Input: part model. Units: mm. Frame: model coordinates. Face numbers are marked on the shaded views. A direction names the side the tool comes from. Coordinates: 2 decimals unless noted, no trailing zeros. Loops run counter-clockwise (first coordinate to the right, second up) from the corner with the lowest first, then second, coordinate; pieces in that order, holes last.
```python
from build123d import *

# Parameters (mm, degrees)
SKETCH1_R                = 50
BOSS_EXTRUDE1_DEPTH      = 129.45
CUT_EXTRUDE1_DEPTH       = 129.45
CUT_EXTRUDE1_DEPTH_BACK  = 129.45
SKETCH3_W                = 73.302623589
SKETCH3_H                = 112.659736925
BOSS_EXTRUDE2_DEPTH      = 10
BOSS_EXTRUDE2_DEPTH_BACK = 10
SKETCH2_R                = 15


with BuildPart() as part:
    # Sketch1 → Boss-Extrude1 (new body)
    with BuildSketch(Plane(origin=(0, 0, 0), x_dir=(0, 0, -1), z_dir=(1, 0, 0))):
        Circle(SKETCH1_R)
    extrude(amount=-BOSS_EXTRUDE1_DEPTH)

    # Sketch3 → Cut-Extrude1 (cut, two sides: drawn at the far end of the back side and taken through both)
    with BuildSketch(Plane(origin=(0, 0, 0), x_dir=(1, 0, 0), z_dir=(0, 1, 0)).offset(-CUT_EXTRUDE1_DEPTH_BACK)):
        with Locations((-96.101311794, -3.115771473)):
            Rectangle(SKETCH3_W, SKETCH3_H)
    extrude(amount=CUT_EXTRUDE1_DEPTH + CUT_EXTRUDE1_DEPTH_BACK, mode=Mode.SUBTRACT)

    # Sketch2 → Boss-Extrude2 (add, two sides: drawn at the far end of the back side and taken through both)
    with BuildSketch(Plane(origin=(0, 0, 0), x_dir=(1, 0, 0), z_dir=(0, 1, 0)).offset(-BOSS_EXTRUDE2_DEPTH_BACK)):
        with BuildLine():
            Line((-129.45, 30), (-59.45, 30))
            Line((-59.45, 30), (-59.45, -30))
            Line((-59.45, -30), (-129.45, -30))
            ThreePointArc((-129.45, -30), (-159.45, 0), (-129.45, 30))
        make_face()
        with Locations(Location((-129.45, 0, 0), (0, 0, 270))):
            Circle(SKETCH2_R, mode=Mode.SUBTRACT)
    extrude(amount=BOSS_EXTRUDE2_DEPTH + BOSS_EXTRUDE2_DEPTH_BACK)


solid = part.part
```
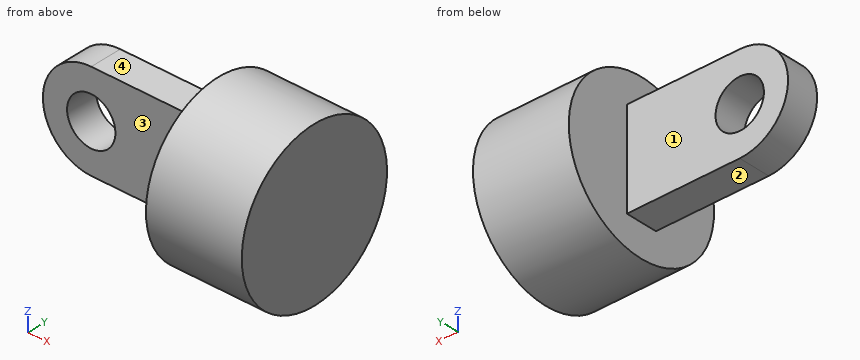
Item 1: Section query C-C (x = -34.5). Output: boundary loops of the cut face in (y, z).
Result:
outline: circle Ø100 at (0, 0)
Item 2: Section query B-B (x = -137). Output: boundary loops of the cut face in (y, z).
Result:
outline: (-10, -29.03) - (10, -29.03) - (10, -12.96) - (-10, -12.96) - close; (-10, 12.96) - (10, 12.96) - (10, 29.03) - (-10, 29.03) - close
Item 3: Reachability of the marked faces 1, 2, 3 and 4 from +Z, -Z, +X, -X, +Y, -Y: full face, straight path, thin tool, end or side. Return the list, or none.
Result:
face 1: +Z, -Z, -X, +Y
face 2: -Z, -X, +Y, -Y
face 3: +Z, -Z, -X, -Y
face 4: +Z, -X, +Y, -Y
Item 4: Section query D-D (z = 23). Output: boundary loops of the cut face in (x, y), then the cut area to 3 significant figures.
Result:
outline: (-148.71, -10) - (-59.45, -10) - (-59.45, -44.4) - (0, -44.4) - (0, 44.4) - (-59.45, 44.4) - (-59.45, 10) - (-148.71, 10) - close
area: 7,060 mm2
Item 5: Line query: L1, parallel to Z at x = -129, y = -3; L2, parallel to X at y = 5.75, z = 0; L3, parallel to X at y = -13, z = 22. Output: solid intervals per line, ascending.
Result:
L1: z = -30 to -14.99, 14.99 to 30
L2: x = -159.45 to -144.45, -114.45 to 0
L3: x = -59.45 to 0
Item 6: Contact query for flat-ended pins moving along their axis: P1, Ø22, axis at x = -99.5, y = -1, coming from the -Z side; P2, Ø10, axis at x = -103.5, y = 0.5, coming from the +Z side; P3, Ø1.5, axis at x = -111.5, z = 12, coming from the +Y side; P4, Ø24, axis at x = -129.45, z = 0, coming from the -Y side. Output: stop coordinate, or through.
Result:
P1: stops at z = -30
P2: stops at z = 30
P3: stops at y = 10
P4: passes through
Item 7: Section query A-A (z = 0). Output: boundary loops of the cut face in (x, y), then the cut area to 4 significant figures.
Result:
outline: (-159.45, -10) - (-144.45, -10) - (-144.45, 10) - (-159.45, 10) - close; (-114.45, -10) - (-59.45, -10) - (-59.45, -50) - (0, -50) - (0, 50) - (-59.45, 50) - (-59.45, 10) - (-114.45, 10) - close
area: 7,345 mm2
